from build123d import *

# Parameters (mm, degrees)
SKETCH1_W           = 66
SKETCH1_H           = 31
SKETCH1_R           = 1.5
BOSS_EXTRUDE1_DEPTH = 1.5
SKETCH2_W           = 14
SKETCH2_H           = 10
BOSS_EXTRUDE2_DEPTH = 2.6
SKETCH3_W           = 6.8
SKETCH3_H           = 7
BOSS_EXTRUDE3_DEPTH = 5
SKETCH4_R           = 2.25
SKETCH4_R_2         = 1.5
BOSS_EXTRUDE4_DEPTH = 0.05
SKETCH5_W           = 5.2
SKETCH5_H           = 10
SKETCH5_W_2         = 3.6
SKETCH5_H_2         = 8.4
BOSS_EXTRUDE5_DEPTH = 10.7
CHAMFER1_SIZE       = 1
FILLET1_R           = 1.5
SKETCH6_R           = 1.5
BOSS_EXTRUDE6_DEPTH = 2
CHAMFER2_SIZE       = 1


with BuildPart() as part:
    # Sketch1 → Boss-Extrude1 (new body)
    with BuildSketch(Plane.XY):
        Rectangle(SKETCH1_W, SKETCH1_H)
        with Locations((30, 12.5)):
            Circle(SKETCH1_R, mode=Mode.SUBTRACT)
        with Locations((30, -12.5)):
            Circle(SKETCH1_R, mode=Mode.SUBTRACT)
        with Locations((-30, -12.5)):
            Circle(SKETCH1_R, mode=Mode.SUBTRACT)
        with Locations((-30, 12.5)):
            Circle(SKETCH1_R, mode=Mode.SUBTRACT)
    extrude(amount=BOSS_EXTRUDE1_DEPTH)

    # Sketch2 → Boss-Extrude2 (add)
    with BuildSketch(Plane.XY.offset(1.5)):
        with Locations((16, -4.5)):
            Rectangle(SKETCH2_W, SKETCH2_H)
    extrude(amount=BOSS_EXTRUDE2_DEPTH)

    # Sketch3 → Boss-Extrude3 (add)
    with BuildSketch(Plane.XY.offset(1.5)):
        with Locations((2.9, -1)):
            Rectangle(SKETCH3_W, SKETCH3_H)
    extrude(amount=BOSS_EXTRUDE3_DEPTH)

    # Sketch4 → Boss-Extrude4 (add)
    with BuildSketch(Plane.XY.offset(1.5)):
        with Locations((-30, -12.5)):
            Circle(SKETCH4_R)
        with Locations((-30, -12.5)):
            Circle(SKETCH4_R_2, mode=Mode.SUBTRACT)
    boss_extrude4 = extrude(amount=BOSS_EXTRUDE4_DEPTH)

    # Mirror1: Boss-Extrude4 across plane
    add(boss_extrude4.mirror(Plane.XY.offset(0.75)))

    # Sketch5 → Boss-Extrude5 (add)
    with BuildSketch(Plane(origin=(0, 0, 0), x_dir=(-1, 0, 0), z_dir=(0, 0, -1))):
        with Locations((22.3, -9)):
            Rectangle(SKETCH5_W, SKETCH5_H)
        with Locations((22.3, -9)):
            Rectangle(SKETCH5_W_2, SKETCH5_H_2, mode=Mode.SUBTRACT)
    extrude(amount=BOSS_EXTRUDE5_DEPTH)

    # Chamfer1
    chamfer1_edges = [part.edges().sort_by_distance(p)[0] for p in [
        (-24.1, -4.8, -5.35),
        (-20.5, -4.8, -5.35),
    ]]
    chamfer(chamfer1_edges, length=CHAMFER1_SIZE)

    # Fillet1
    fillet1_edges = [part.edges().sort_by_distance(p)[0] for p in [
        (-24.9, -4, -5.35),
        (-19.7, -4, -5.35),
    ]]
    fillet(fillet1_edges, radius=FILLET1_R)

    # Sketch6 → Boss-Extrude6 (add)
    with BuildSketch(Plane(origin=(0, 0, 0), x_dir=(-1, 0, 0), z_dir=(0, 0, -1))):
        with Locations((16, 12.5)):
            Circle(SKETCH6_R)
        with Locations((22, 12.5)):
            Circle(SKETCH6_R)
    extrude(amount=BOSS_EXTRUDE6_DEPTH)

    # Chamfer2
    chamfer2_edges = [part.edges().sort_by_distance(p)[0] for p in [
        (-14.5, 12.5, -2),
        (-20.5, 12.5, -2),
    ]]
    chamfer(chamfer2_edges, length=CHAMFER2_SIZE)


solid = part.part
The model under review builds one solid part; all positions refer to its coordinate system, in mm. A direction names the side the tool comes from. Coordinates: 2 decimals unless noted, no trailing zeros. Order: outer loops, then holes, each group sorted by start corner. A loop starts at its lowest first (then second) coordinate and runs counter-clockwise, first axis right, second up. Notation, with made-up numbers: (0, 70) -> (58, 70) arc R22 cw to (58, 96) -> close; hole circle Ø4 at (51.25, 21.5). An arc over 180 degrees is marked (long way). Answer in a Markdown table with one row per item.
(1) Insertion check: pin 1 (2.5 mm diameter, centred on x = 1.5, z = 5, fed in from +Y); pin 2 (4 mm diameter, centred on y = -9, z = -7, fed in from +X); pin 3 (4 mm diameter, centred on y = -2.5, z = -8, fed in from -X); pin 4 (5.5 mm diameter, centred on y = -2, z = 3.5, fed in from -X). Each pin has a flat end and moves straight along its axis. Give the tip position at first contact, or say it passes through.
Answers:
| item | result |
|---|---|
| pin 1 | y = 2.5 |
| pin 2 | x = -19.7 |
| pin 3 | x = -24.52 |
| pin 4 | x = -33 |
(2) Wall thickness on line 1 along Y through (x, z) = (30, 1); line 2 along X through (y, z) = (-10.5, -7); line 3 along Z through (x, y) = (-28.5, 9.5): over which ranges is each line inside the solid? List them lowest first.
Answers:
| item | result |
|---|---|
| line 1 | -15.5 to -14, -11 to 11, 14 to 15.5 |
| line 2 | -24.9 to -24.1, -20.5 to -19.7 |
| line 3 | 0 to 1.5 |
(3) Consider section B-B (z = -6). Write out the cut boundary in (x, y).
Answers:
| item | result |
|---|---|
| outline | (-24.9, -14) -> (-19.7, -14) -> (-19.7, -5.5) arc R1.5 ccw to (-21.2, -4) -> (-23.4, -4) arc R1.5 ccw to (-24.9, -5.5) -> close; hole (-24.1, -13.2) -> (-20.5, -13.2) -> (-20.5, -5.8) -> (-21.5, -4.8) -> (-23.1, -4.8) -> (-24.1, -5.8) -> close |
(4) Machinability: for faces 5 (the flat face through (-22, -14, -5)), 6 (the flat face through (-0.5, -1, 4)), 7 (the cylindrical face through (-20.5, 12.57, -0.49)), which of the approach directions +Z, -Z, +X, -X, +Y, -Y give a long, thin tool a straight path to every point of the face, cutting with its end or side? Answer none if there is none.
Answers:
| item | result |
|---|---|
| face 5 | -Z, +X, -X, -Y |
| face 6 | +Z, -X, +Y, -Y |
| face 7 | -Z |
(5) Consider section D-D (x = 21). Write out the cut boundary in (y, z), plus the area to 3 significant figures.
Answers:
| item | result |
|---|---|
| outline | (-15.5, 0) -> (15.5, 0) -> (15.5, 1.5) -> (0.5, 1.5) -> (0.5, 4.1) -> (-9.5, 4.1) -> (-9.5, 1.5) -> (-15.5, 1.5) -> close |
| area | 72.5 mm² |
(6) Consider section A-A (x = 30). Write out the cut boundary in (y, z), plus the area to 3 significant figures.
Answers:
| item | result |
|---|---|
| outline | (-15.5, 0) -> (-14, 0) -> (-14, 1.5) -> (-15.5, 1.5) -> close; (-11, 0) -> (11, 0) -> (11, 1.5) -> (-11, 1.5) -> close; (14, 0) -> (15.5, 0) -> (15.5, 1.5) -> (14, 1.5) -> close |
| area | 37.5 mm² |
(7) Consider section C-C (y = -1). Write out the cut boundary in (x, z), plus the area to 3 significant figures.
Answers:
| item | result |
|---|---|
| outline | (-33, 0) -> (33, 0) -> (33, 1.5) -> (23, 1.5) -> (23, 4.1) -> (9, 4.1) -> (9, 1.5) -> (6.3, 1.5) -> (6.3, 6.5) -> (-0.5, 6.5) -> (-0.5, 1.5) -> (-33, 1.5) -> close |
| area | 169 mm² |
(8) The part is to be moulded in two halves that separate along X. For faces 1 (the cylindrical face through (-31.5, -12.43, 0.76)), 2 (the flat face through (23, -5, 3)), 3 (the flat face through (-24.6, -8.9, -10.7)), 4 (the cylindrical face through (-14.5, 12.57, -0.49)), say which applies: +X half, -X half, draft (parallel to the pull), parting line (faces both ways), or undercut.
Answers:
| item | result |
|---|---|
| face 1 | undercut |
| face 2 | +X half |
| face 3 | draft |
| face 4 | undercut |
